Geometry check sheet. Reference: the model listing, model coordinates, mm. A direction names the side the tool comes from. Give positions to 0.01 mm unless a question says otherwise; leave off trailing zeros. Loops run counter-clockwise (first coordinate to the right, second up) from the corner with the lowest first, then second, coordinate; pieces in that order, holes last. Notation, with made-up numbers: (69.5, 63.25) - (92.5, 63.25) arc R16 cw to (92.5, 85.25) - close; hole circle Ø2 at (62.5, -21). An arc over 180 degrees is marked (long way). One line per question, with ' | ' between items. Start each with the question number.
Autodesk Fusion 360 part; units mm, degrees
sketch "Sketch1" plane through (0, 0, 0) normal (0, 0, 1) x (1, 0, 0)
  line L0 (11.35, 9) -> (-11.35, 9) construction
  line L1 (-11.35, 9) -> (-11.35, -9) construction
  line L2 (-11.35, -9) -> (11.35, -9) construction
  line L3 (11.35, -9) -> (11.35, 9) construction
  line L4 (11.35, 9) -> (-11.35, -9) construction
  line L5 (-11.35, 9) -> (11.35, -9) construction
  line L6 (-8.75, 8) -> (8.75, 8)
  line L7 (8.75, 8) -> (8.75, -5.4)
  line L8 (8.75, -5.4) -> (-8.75, -5.4)
  line L9 (-8.75, -5.4) -> (-8.75, 8)
  circle A0 centre (0, 0) radius 3.5
  line L10 (2.4, -0.6) -> (-2.4, -0.6)
  line L11 (-2.4, -0.6) -> (-2.4, 0.6)
  line L12 (-2.4, 0.6) -> (2.4, 0.6)
  line L13 (2.4, 0.6) -> (2.4, -0.6)
  line L14 (2.4, -0.6) -> (-2.4, 0.6) construction
  line L15 (-2.4, -0.6) -> (2.4, 0.6) construction
  line L16 (0.6, -2.4) -> (-0.6, -2.4)
  line L17 (-0.6, -2.4) -> (-0.6, 2.4)
  line L18 (-0.6, 2.4) -> (0.6, 2.4)
  line L19 (0.6, 2.4) -> (0.6, -2.4)
  line L20 (0.6, -2.4) -> (-0.6, 2.4) construction
  line L21 (-0.6, -2.4) -> (0.6, 2.4) construction
  line L22 (-0.6, 2.4) -> (-2.5475, 2.4)
  line L23 (0.6, 2.4) -> (2.5475, 2.4)
  line L24 (-0.6, -2.4) -> (-2.5475, -2.4)
  line L25 (0.6, -2.4) -> (2.5475, -2.4)
  dimension "d1" = 22.7
  dimension "d2" = 18
  dimension "d3" = 3.6
  dimension "d4" = 1
  dimension "d5" = 2.6
  dimension "d6" = 2.6
  dimension "d7" = 7
  dimension "d8" = 4.8
  dimension "d9" = 1.2
  dimension "d10" = 1.2
  dimension "d11" = 4.8
extrude "Extrude1" add sketch "Sketch1" along normal blind 0.6 contours L6 L7 L8 L9 | A0 L10 L12 L13 L19 L23 L25 | A0 L18 L22 L23 | A0 L16 L24 L25 | A0 L10 L11 L12 L17 L22 L24 | L12 L17 L18 L19 | L10 L16 L17 L19 | L10 L12 L17 L19 | L10 L12 L13 L19 | L10 L11 L12 L17
extrude "Extrude2" add sketch "Sketch1" along normal blind 4 contours A0 L10 L12 L13 L19 L23 L25 | A0 L10 L11 L12 L17 L22 L24
fillet "Fillet1" radius 1 6 edges at (-1.5738, -2.4, 0.6) (-3.5, 0, 0.6) (1.5738, -2.4, 0.6) (3.5, 0, 0.6) (1.5738, 2.4, 0.6) (-1.5738, 2.4, 0.6)
fillet "Fillet1" radius 0.5 4 edges at (8.75, 8, 0.3) (-8.75, 8, 0.3) (8.75, -5.4, 0.3) (-8.75, -5.4, 0.3)
chamfer "Chamfer1" distance 0.4 angle 45 20 edges at (-8.6036, 7.8536, 0) (0, 8, 0) (8.6036, 7.8536, 0) (8.75, 1.3, 0) (8.6036, -5.2536, 0) (0, -5.4, 0) (-8.6036, -5.2536, 0) (-8.75, 1.3, 0) (-0.6, 1.5, 4) (-1.5, 0.6, 4) (-2.4, 0, 4) (-1.5, -0.6, 4) (-0.6, -1.5, 4) (0.6, -1.5, 4) (1.5, -0.6, 4) (2.4, 0, 4) (1.5, 0.6, 4) (0.6, 1.5, 4) (3.5, 0, 4) (-3.5, 0, 4)
(1) Depth check by flat-ended pin: pin 1 Ø0.6 at (x, z) = (1.5, 3) entering from -Y; pin 2 Ø1.4 at (y, z) = (-2, 2) entering from +X; pin 3 Ø0.6 at (y, z) = (0, 2) entering from -X. Enter the tip coordinate at first touch or a pass-through.
(2) Section check B-B, the plane y = 0. Record the boundary of the cut face in (x, z), and give its area (3 significant figures).
(3) Section check D-D, the plane x = -5. Record the boundary of the cut face in (y, z).
(4) Material ranges on line 1 (Z direction, x = 8.25, y = 3.25); line 2 (X direction, y = -0.75, z = 1.15); line 3 (X direction, y = -1, z = 2.95), recorded low to high.
(5) Section check C-C, the plane x = -1.5. Record the boundary of the cut face in (y, z), and give its area (3 significant figures).
(6) Tool access check on faces 1 (the face through (2, 2.4, 3)), 2 (the face through (0, 1, 0)), 3 (the face through (-3.5, 0, 2.6)), 4 (the face through (-2, -2.4, 3)), 5 (the face through (-2, 0.6, 2)). Record the directions out of +Z, -Z, +X, -X, +Y, -Y that give a thin tool (end or side, any length) a straight path to the whole face; none if there is none.
(7) Mould release check, pull along Y, two halves, no side actions. Record for faces 6 (the face through (2.4, 0, 2)), 7 (the face through (3.5, 0, 2.6)), 8 (the face through (-0.6, 2, 2)): pulls with the +Y half, pulls with the -Y half, needs draft (parallel to the pull), parting line crosses it, or undercut.
(8) Section check A-A, the plane z = 2.8. Record the boundary of the cut face in (x, y), and give its area (3 significant figures).
Numbers:
1) pin 1: y = -2.4 | pin 2: x = 3.25 | pin 3: x = -3.5
2) outline: (-8.75, 0.4) - (-8.35, 0) - (8.35, 0) - (8.75, 0.4) - (8.75, 0.6) - (4.5, 0.6) arc R1 cw to (3.5, 1.6) - (3.5, 3.6) - (3.1, 4) - (2.8, 4) - (2.4, 3.6) - (2.4, 0.6) - (-2.4, 0.6) - (-2.4, 3.6) - (-2.8, 4) - (-3.1, 4) - (-3.5, 3.6) - (-3.5, 1.6) arc R1 cw to (-4.5, 0.6) - (-8.75, 0.6) - close | area: 17.9 mm^2
3) outline: (-5.4, 0.4) - (-5, 0) - (7.6, 0) - (8, 0.4) - (8, 0.6) - (-5.4, 0.6) - close
4) line 1: 0 to 0.6 | line 2: -3.53 to -0.6, 0.6 to 3.53 | line 3: -3.35 to -0.6, 0.6 to 3.35
5) outline: (-5.4, 0.4) - (-5, 0) - (7.6, 0) - (8, 0.4) - (8, 0.6) - (3.4, 0.6) arc R1 cw to (2.4, 1.6) - (2.4, 4) - (1, 4) - (0.6, 3.6) - (0.6, 0.6) - (-0.6, 0.6) - (-0.6, 3.6) - (-1, 4) - (-2.4, 4) - (-2.4, 1.6) arc R1 cw to (-3.4, 0.6) - (-5.4, 0.6) - close | area: 20.4 mm^2
6) face 1: +Z, +X, -X, +Y | face 2: -Z, +X, -X, +Y, -Y | face 3: +Z, -X | face 4: +Z, +X, -X, -Y | face 5: +Z
7) face 6: undercut | face 7: parting line crosses it | face 8: needs draft
8) outline: (-2.55, -2.4) - (-0.6, -2.4) - (-0.6, -0.6) - (-2.4, -0.6) - (-2.4, 0.6) - (-0.6, 0.6) - (-0.6, 2.4) - (-2.55, 2.4) arc R3.5 ccw to start; (0.6, -2.4) - (2.55, -2.4) arc R3.5 ccw to (2.55, 2.4) - (0.6, 2.4) - (0.6, 0.6) - (2.4, 0.6) - (2.4, -0.6) - (0.6, -0.6) - close | area: 20.7 mm^2
